The figure shows three views and two pictorial views of one solid part (mm, origin at its lowest corner). Answer the questions. A direction names the side the tool comes from. Round coordinates to 2 decimals unless told otherwise and drop trailing zeros. Order: outer loops, then holes, each group sorted by start corner. A loop starts at its lowest first (then second) coordinate and runs counter-clockwise, first axis right, second up. Notation, with made-up numbers: (1.5, 56.25) -> (27.5, 56.25) arc R25 ccw to (27.5, 75.25) -> close; hole circle Ø6 at (25, 25.5). An arc over 180 degrees is marked (long way). Return JSON: item names as keys, results as strings. Group by question number.
(1) The part is cut by section A-A (x = 2.75). Determine the outline of the cut face in (y, z), plus the area to 3 significant figures.
(2) The part is cut by section B-B (y = 6). Determine the outline of the cut face in (x, z).
(3) Each of these flat-tipped pins is pushed along its axis until it touches: pin 1 (2 mm diameter, centred on y = 3.5, z = 1.5, fed in from -X); pin 2 (2.5 mm diameter, centred on x = 4, y = 6.5, fed in from +Z); pin 3 (0.7 mm diameter, centred on x = 3, y = 5.5, fed in from -Z); pin 4 (1 mm diameter, centred on x = 1.5, z = 4.5, fed in from +Y). Where does it stop, or does it pass through?
(4) Consider line 1 (Y direction, x = 5.75, z = 2.8); line 2 (Z direction, x = 4, y = 3.5); line 3 (X direction, y = 4, z = 3.35). Determine where each line is inside the solid, lowest interval first. Write a range as [from, to].
(5) The part is cut by section D-D (x = 1). Determine the outline of the cut face in (y, z), plus the area to 3 significant figures.
(6) The part is cut by section C-C (z = 4.1). Determine the outline of the cut face in (x, y).
(7) Which of the six approach directions +Z, -Z, +X, -X, +Y, -Y give full straight-line access (tool end or side, diameter ignored) to the marked faces 1, 2, 3, 4 and 5?
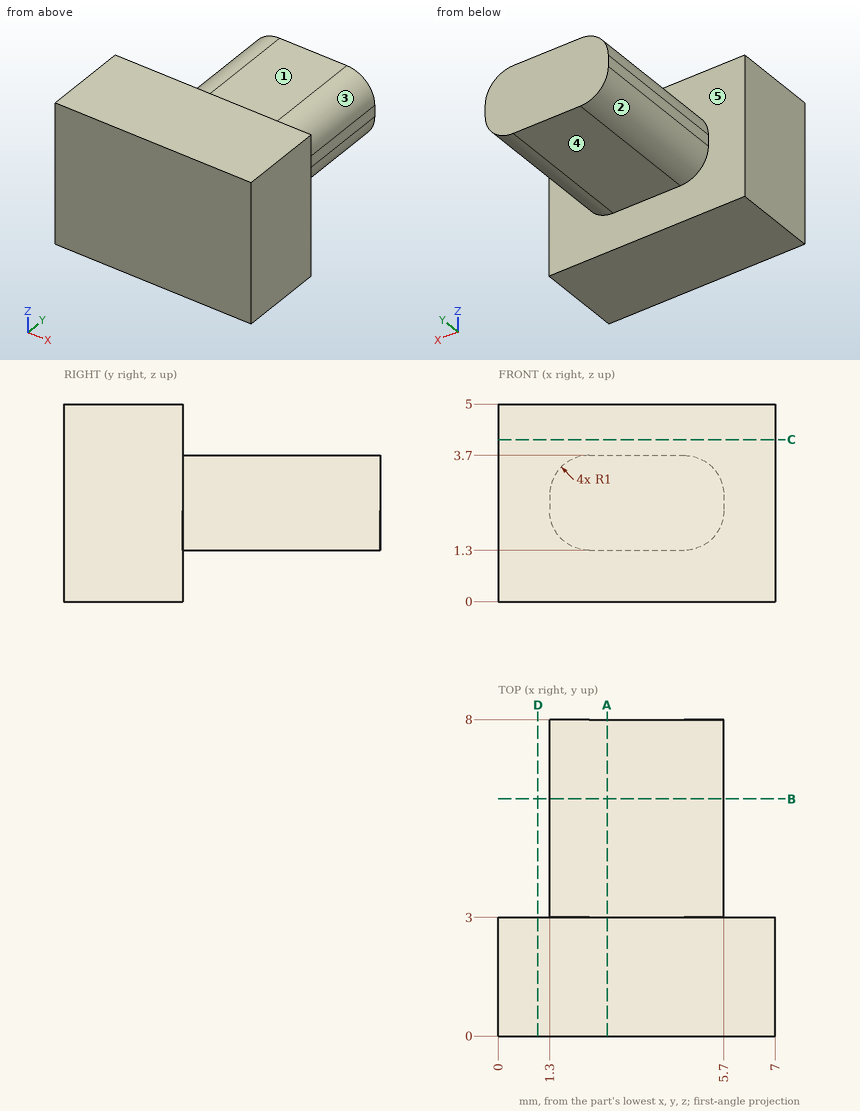
Answer below:
{
 "1": {"outline": "(0, 0) -> (3, 0) -> (3, 1.3) -> (8, 1.3) -> (8, 3.7) -> (3, 3.7) -> (3, 5) -> (0, 5) -> close", "area": "27.0 mm²"},
 "2": {"outline": "(1.3, 2.3) arc R1 ccw to (2.3, 1.3) -> (4.7, 1.3) arc R1 ccw to (5.7, 2.3) -> (5.7, 2.7) arc R1 ccw to (4.7, 3.7) -> (2.3, 3.7) arc R1 ccw to (1.3, 2.7) -> close"},
 "3": {"pin 1": "stops at x = 0", "pin 2": "stops at z = 3.7", "pin 3": "stops at z = 1.3", "pin 4": "stops at y = 3"},
 "4": {"line 1": "y = [0, 3]", "line 2": "z = [1.3, 3.7]", "line 3": "x = [1.54, 5.46]"},
 "5": {"outline": "(0, 0) -> (3, 0) -> (3, 5) -> (0, 5) -> close", "area": "15.0 mm²"},
 "6": {"outline": "(0, 0) -> (7, 0) -> (7, 3) -> (0, 3) -> close"},
 "7": {"face 1": "+Z, +X, -X, +Y", "face 2": "-Z, -X, +Y", "face 3": "+Z, +X, +Y", "face 4": "-Z, +X, -X, +Y", "face 5": "+Y"}
}
